from build123d import *

# Parameters (mm, degrees)
F1_DEPTH = 2.54
F2_SIZE  = 2.53999


# Not quite as in the source:
# - a fillet or chamfer is up to 0.001 mm smaller than in the source, because OpenCascade refuses the exact size


with BuildPart() as f1:
    # F0 (on Front) → F1 (new body)
    with BuildSketch(Plane.XZ):
        with BuildLine():
            Line((-12.3092299327, 19.36452277), (-64.2481818795, 19.36452277))
            ThreePointArc((-64.2481818795, 19.36452277), (-48.7050050326, 13.9320089842), (-39.9299450219, 0))
            ThreePointArc((-39.9299450219, 0), (-24.1018123493, -1.5321631259), (-12.0090059936, -11.8588926271))
            ThreePointArc((-12.0090059936, -11.8588926271), (-6.881876251, -7.2071480524), (0, -6.4548407681))
            ThreePointArc((0, -6.4548407681), (6.881876251, -7.2071480524), (12.0090059936, -11.8588926271))
            ThreePointArc((12.0090059936, -11.8588926271), (24.1018123493, -1.5321631259), (39.9299450219, 0))
            ThreePointArc((39.9299450219, 0), (48.7050050326, 13.9320089842), (64.2481818795, 19.36452277))
            Line((64.2481818795, 19.36452277), (12.3092299327, 19.36452277))
            Line((12.3092299327, 19.36452277), (9.3069793656, 9.7573176026))
            Line((9.3069793656, 9.7573176026), (9.3069793656, 26.2697003782))
            Line((9.3069793656, 26.2697003782), (5.4040518589, 22.3667733371))
            Line((5.4040518589, 22.3667733371), (0, 22.3667733371))
            Line((0, 22.3667733371), (-5.4040518589, 22.3667733371))
            Line((-5.4040518589, 22.3667733371), (-9.3069793656, 26.2697003782))
            Line((-9.3069793656, 26.2697003782), (-9.3069793656, 9.7573176026))
            Line((-9.3069793656, 9.7573176026), (-12.3092299327, 19.36452277))
        make_face()
    extrude(amount=F1_DEPTH)

    # F2 (size 2.54 in the source; OpenCascade refuses exactly that, so slightly less here)
    f2_edges = [f1.edges().sort_by_distance(p)[0] for p in [
        (-38.278706, -2.54, 19.364523),
        (38.278706, -2.54, 19.364523),
        (48.705005, -2.54, 13.932009),
        (24.101812, -2.54, -1.532163),
        (6.881876, -2.54, -7.207148),
        (-6.881876, -2.54, -7.207148),
        (-24.101812, -2.54, -1.532163),
        (-48.705005, -2.54, 13.932009),
        (-7.355516, -2.54, 24.318237),
        (0, -2.54, 22.366773),
        (7.355516, -2.54, 24.318237),
    ]]
    chamfer(f2_edges, length=F2_SIZE)


solid = f1.part
The listing builds one solid part. Answer for the finished solid, in the listing's coordinates (mm). A direction names the side the tool comes from. Coordinates: 2 decimals unless noted, no trailing zeros. Write each loop counter-clockwise with the first axis right and the second up, starting at its lowest first coordinate (ties: lowest second). Pieces come first, ordered by that corner, then holes. Notation, with made-up numbers: M 39.5,-11 L 80.5,-11 A16 cw 80.5,4 Z; hole C 57,-19.5 d8. An arc over 180 degrees is marked long. Put each result on its own line as item: value. Start each with the question number.
1. Which of the six approach directions +Z, -Z, +X, -X, +Y, -Y give full straight-line access (tool end or side, diameter ignored) to faces 1 (the conical face through (-45.61, -0.72, 12.07)), 2 (the flat face through (-7.86, -1.29, 23))?
2. For a pull along X with two mould halves and no side action, classify faces 3 (the conical face through (45.3, -0.7, 11.7)), 4 (the conical face through (-5.8, -1.01, -5.73)), 5 (the flat face through (-1, -2.54, 8)) as pulls with the +X half, pulls with the -X half, needs draft (parallel to the pull), parting line crosses it, or undercut.
3. A cutting plane is placed at B-B on y = -0.6. Write down the section's boundary in (x, z), then the cut area to 3 significant figures.
4. Consider line 1 (X direction, y = -0.8, z = 13); line 2 (X direction, y = -1.45, z = 17); line 3 (X direction, y = -2.4, z = -7). Determine where each line is inside the solid, lowest interval first. Write a range as from..to.
5. Flat-ended cylindrical pins translate along their axes: P1, Ø8, axis at x = -5.5, z = 0, coming from the +Y side; P2, Ø1.5, axis at y = -0.5, z = 2, coming from the -X side. Find the tip coordinate at first contact, or state that the pin passes through.
6. A cutting plane is placed at C-C on z = 11.5. Count the separate pieces of the cut face and the enclosed holes in it, then the cut area to 3 significant figures.
Resolved:
1. face 1: -Z, -X, -Y
1. face 2: +Z, -Y
2. face 3: pulls with the +X half
2. face 4: undercut
2. face 5: needs draft
3. outline: M -56.51,18.76 A25.55 cw -39.48,0.7 A27.07 cw -12.02,-10.75 A11.81 cw 0,-5.84 A11.81 cw 12.02,-10.75 A27.07 cw 39.48,0.7 A25.55 cw 56.51,18.76 L 12.12,18.76 L 9.31,9.76 L 9.31,25.42 L 5.65,21.77 L -5.65,21.77 L -9.31,25.42 L -9.31,9.76 L -12.12,18.76 Z
3. area: 1,990 mm2
4. line 1: x = -46.42..-10.32, -9.31..9.31, 10.32..46.42
4. line 2: x = -50.58..-11.57, -9.31..9.31, 11.57..50.58
4. line 3: x = -12.62..-11.03, 11.03..12.62
5. P1: stops at y = 0
5. P2: stops at x = -40.66
6. separate pieces: 3
6. enclosed holes: 0
6. area: 223 mm2
